Job drawing, mm, ordinate dimensions from the low corner. One solid piece. Give positions to 0.01 mm unless a question says otherwise; leave off trailing zeros. Order: outer loops, then holes, each group sorted by start corner. A loop starts at its lowest first (then second) coordinate and runs counter-clockwise, first axis right, second up. Notation, with made-up numbers: (52, 21) -> (99, 21) arc R19 cw to (99, 48) -> close; hole circle Ø1 at (34, 66.25). An arc over 180 degrees is marked (long way). Use CSV: the item, a comma, the result in double quotes. Start each with the question number.
1. Wall check: line 1 (Y direction, x = 16, z = 15.5); line 2 (X direction, y = 16.25, z = 18); line 3 (X direction, y = 11.5, z = 23.75). Give the ranges that are in metal, low to high. Write a range as from..to.
2. Drop flat-ended pins along their axis: pin 1 (5 mm diameter, centred on x = 4.5, z = 18.5, fed in from -Y); pin 2 (4 mm diameter, centred on x = 17.5, z = 21.5, fed in from +Y); pin 3 (3 mm diameter, centred on x = 13, z = 7, fed in from +Y). Give the stop position or say it passes through.
3. Cut at D-D on z = 12.5. List the corners of the cut face in (x, y), then the cut area to 3 significant figures.
4. Pull direction Y, two halves, no side cores. Call the marked faces 1 and 2: released by +Y, released by -Y, zero draft, split by the parting line, or undercut.
5. Cut at C-C on z = 5. List the corners of the cut face in (x, y).
6. Cut at A-A on x = 10. List the corners of the cut face in (y, z), then the cut area to 3 significant figures.
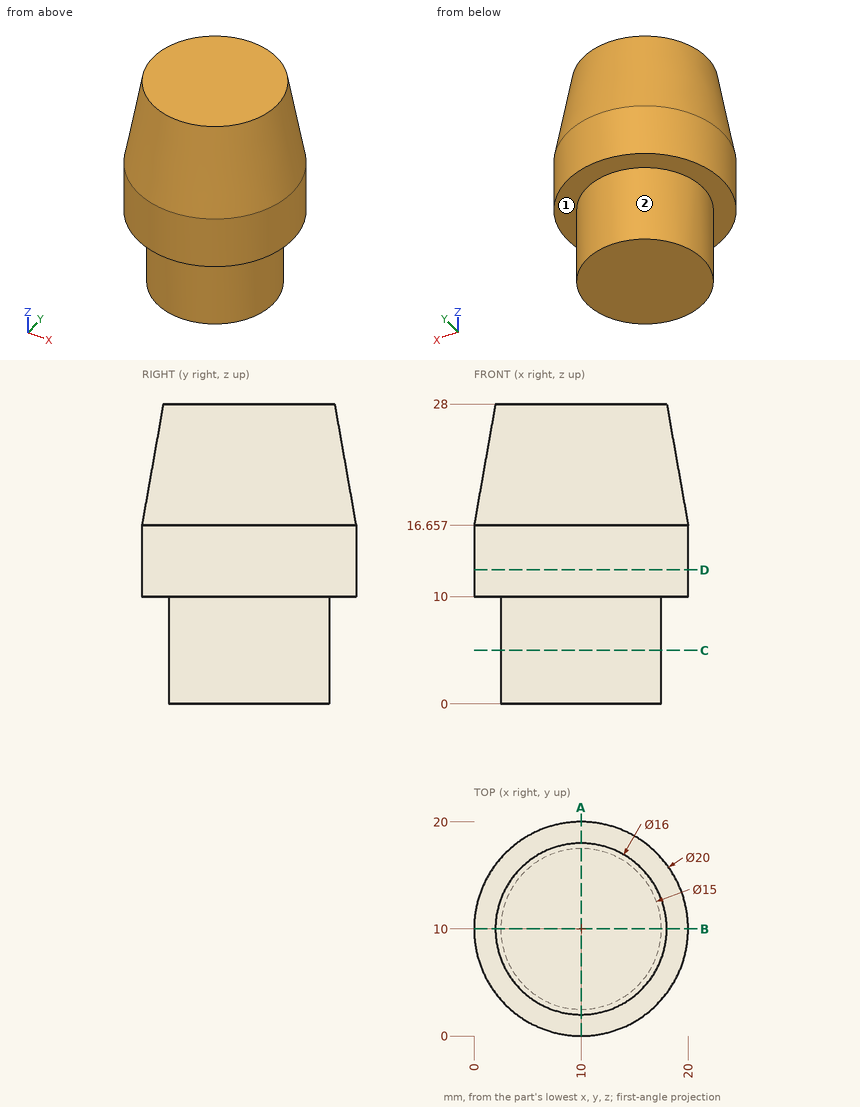
Verdict:
1,line 1,"2..18"
1,line 2,"2.5..17.5"
1,line 3,"1.38..18.62"
2,pin 1,"y = 0.68"
2,pin 2,"y = 17.37"
2,pin 3,"y = 17.35"
3,outline,"circle Ø20 at (10, 10)"
3,area,"314 mm^2"
4,face 1,"zero draft"
4,face 2,"split by the parting line"
5,outline,"circle Ø15 at (10, 10)"
6,outline,"(0, 10) -> (2.5, 10) -> (2.5, 0) -> (17.5, 0) -> (17.5, 10) -> (20, 10) -> (20, 16.66) -> (18, 28) -> (2, 28) -> (0, 16.66) -> close"
6,area,"487 mm^2"
